Model file for the job. Use its own axes, mm. A direction names the side the tool comes from. Coordinates: 2 decimals unless noted, no trailing zeros. Write each loop counter-clockwise with the first axis right and the second up, starting at its lowest first coordinate (ties: lowest second). Pieces come first, ordered by that corner, then holes. Notation, with made-up numbers: M 61.5,71.25 L 96.5,71.25 A34 ccw 96.5,109.25 Z; hole C -22.75,52.25 d2. An arc over 180 degrees is marked long. One line per question, with ' | ' between items. Start each with the question number.
(1) Cut at B-B (z = -166.5). Write the cut outline in (x, y).
(2) Wall check: probe 1 along Y at (x, z) = (41.5, -167); probe 2 along X at (y, z) = (3.5, -165.5); probe 3 along X at (y, z) = (6, -170.5). Give the ranges that are in metal, low to high.
(3) Cut at A-A (y = 4.25). Write the cut outline in (x, z).
(4) Flat gauge pins, fed straight in: pin 1 Ø5 at (x, z) = (-35, -175) entering from -Y; pin 2 Ø7.5 at (x, z) = (-17.5, -169) entering from +Y. Where does each tip first touch, or does it go through?
(5) Cut at C-C (x = 7.5). Write the cut outline in (y, z), plus the area to 3 significant figures.
(6) Two-plate mould, pull along Z, no slides. Class faces 6 (the face through (41.74, 3.48, -169.05)), 7 (the face through (42.65, -2.46, -171.58)), 8 (the face through (42, -5, -173)): +Z half, -Z half, draft (parallel to the pull), parting line (faces both ways), or undercut.
(7) Cut at D-D (y = -2.25). Write the cut outline in (x, z).
(8) Tool access for faces 1 (the face through (0.64, 3.45, -181.21)), 2 (the face through (-38.685, 0.986, -168.419)), 3 (the face through (-41.498, -2.465, -171.578)), 4 (the face through (-42, -5, -173)), 5 (the face through (-41.692, 3.479, -168.919)): list every direction of +Z, -Z, +X, -X, +Y, -Y with a clear straight run to the whole face (end or side of a thin tool).
from build123d import *

# Parameters (mm, degrees)
BOSS_EXTRUDE4_DEPTH = 2
BOSS_EXTRUDE5_DEPTH = 3
BOSS_EXTRUDE6_DEPTH = 2
SKETCH7_R           = 1.5
BOSS_EXTRUDE7_DEPTH = 5


with BuildPart() as part:
    # Sketch2 → Boss-Extrude4 (new body)
    with BuildSketch(Plane(origin=(0, 0, 0), x_dir=(1, 0, 0), z_dir=(0, 1, 0))):
        with BuildLine():
            Line((-44.292533925, 163.999092012), (-38.292533925, 163.999092012))
            Line((-38.292533925, 163.999092012), (-39.089453392, 172.963740324))
            ThreePointArc((-39.089453392, 172.963740324), (0, 177.325804195), (39.089453392, 172.963740324))
            Line((39.089453392, 172.963740324), (38.292533925, 163.999092012))
            Line((38.292533925, 163.999092012), (44.292533925, 163.999092012))
            Line((44.292533925, 163.999092012), (45.310819911, 175.453920411))
            ThreePointArc((45.310819911, 175.453920411), (0, 181.210233123), (-45.310819911, 175.453920411))
            Line((-45.310819911, 175.453920411), (-44.292533925, 163.999092012))
        make_face()
    extrude(amount=BOSS_EXTRUDE4_DEPTH)

    # Sketch5 → Boss-Extrude5 (add)
    with BuildSketch(Plane(origin=(0, 2, 0), x_dir=(1, 0, 0), z_dir=(0, 1, 0))):
        with BuildLine():
            Line((-41.292533925, 163.999092012), (-42.102735456, 173.978043635))
            ThreePointArc((-42.102735456, 173.978043635), (0.038720573, 178.999995812), (42.178, 173.959812359))
            Line((42.178, 173.959812359), (41.292533925, 163.999092012))
            Line((41.292533925, 163.999092012), (44.292533925, 163.999092012))
            Line((44.292533925, 163.999092012), (45.310819911, 175.453920411))
            ThreePointArc((45.310819911, 175.453920411), (0, 181.210233123), (-45.310819911, 175.453920411))
            Line((-45.310819911, 175.453920411), (-44.292533925, 163.999092012))
            Line((-44.292533925, 163.999092012), (-41.292533925, 163.999092012))
        make_face()
    extrude(amount=BOSS_EXTRUDE5_DEPTH)

    # Sketch6 → Boss-Extrude6 (add)
    with BuildSketch(Plane(origin=(0, 5, 0), x_dir=(1, 0, 0), z_dir=(0, 1, 0))):
        with BuildLine():
            Line((-44.292533925, 163.999092012), (-38.292533925, 163.999092012))
            Line((-38.292533925, 163.999092012), (-39.089453392, 172.963740324))
            ThreePointArc((-39.089453392, 172.963740324), (0, 177.325804195), (39.089453392, 172.963740324))
            Line((39.089453392, 172.963740324), (38.292533925, 163.999092012))
            Line((38.292533925, 163.999092012), (44.292533925, 163.999092012))
            Line((44.292533925, 163.999092012), (45.310819911, 175.453920411))
            ThreePointArc((45.310819911, 175.453920411), (0, 181.210233123), (-45.310819911, 175.453920411))
            Line((-45.310819911, 175.453920411), (-44.292533925, 163.999092012))
        make_face()
    extrude(amount=BOSS_EXTRUDE6_DEPTH)

    # Sketch7 → Boss-Extrude7 (add)
    with BuildSketch(Plane.XZ):
        with Locations(Location((-42.072341363, -172.963740324, 0), (0, 0, 90))):
            Circle(SKETCH7_R)
        with Locations(Location((42.072341363, -172.963740324, 0), (0, 0, 90))):
            Circle(SKETCH7_R)
    extrude(amount=BOSS_EXTRUDE7_DEPTH)


solid = part.part
Filled in:
1) outline: M -44.51,0 L -38.51,0 L -38.51,2 L -41.5,2 L -41.5,5 L -38.51,5 L -38.51,7 L -44.51,7 Z; M 38.51,0 L 44.51,0 L 44.51,7 L 38.51,7 L 38.51,5 L 41.51,5 L 41.51,2 L 38.51,2 Z
2) probe 1: 0 to 2, 5 to 7 | probe 2: -44.43 to -41.41, 41.43 to 44.43 | probe 3: -44.87 to -38.87, 38.87 to 44.87
3) outline: M -45.31,-175.45 A181.21 ccw 45.31,-175.45 L 44.29,-164 L 41.29,-164 L 42.18,-173.96 A179 cw -42.1,-173.98 L -41.29,-164 L -44.29,-164 Z
4) pin 1: y = 0 | pin 2: through
5) outline: M 0,-181.05 L 7,-181.05 L 7,-177.17 L 5,-177.17 L 5,-178.84 L 2,-178.84 L 2,-177.17 L 0,-177.17 Z | area: 22.2 mm²
6) face 6: undercut | face 7: parting line | face 8: draft
7) outline: C -42.07,-172.96 d3; C 42.07,-172.96 d3
8) face 1: -Z, +Y, -Y | face 2: +Y, -Y | face 3: -Y | face 4: +Z, -Z, +X, -X, -Y | face 5: none
